Design review of the part built by this model. Coordinates are the model's own, in mm. A direction names the side the tool comes from. Give positions to 0.01 mm unless a question says otherwise; leave off trailing zeros. Write each loop counter-clockwise with the first axis right and the second up, starting at its lowest first coordinate (ties: lowest second). Pieces come first, ordered by that corner, then holes. Notation, with made-up numbers: (-19, 48) -> (-5, 48) arc R31 cw to (-5, 73) -> close; hole circle Ø9 at (7.5, 42). An arc over 180 degrees is marked (long way). Use CSV: the item, a comma, the result in double quotes.
```python
from build123d import *

# Parameters (mm, degrees)
F0_W      = 100
F0_H      = 63
F1_DEPTH  = 50
F3_DEPTH  = 50.001
F4_W      = 40
F4_H      = 15
F5_DEPTH  = 50.001
F7_DEPTH  = 9
F8_R      = 5
F9_DEPTH  = 41.001
F10_W     = 12
F10_H     = 10
F10_H_2   = 40
F11_DEPTH = 63.001
F13_DEPTH = 187
F15_DEPTH = 100.001
F16_R     = 25
F17_DEPTH = 18
F18_R     = 10
F19_DEPTH = 5
F22_DEPTH = 42
F20_R     = 25
F23_DEPTH = 8
F25_DEPTH = 8
F26_W     = 40
F26_H     = 9
F27_DEPTH = 8.001
F28_R     = 5
F29_DEPTH = 63.001


# Not quite as in the source:
# - an extrude ends at something that could not be found from the text; its depth is read off the source's solid


with BuildPart() as f1:
    # F0 (on Right) → F1 (new body)
    with BuildSketch(Plane.YZ):
        with Locations((50, 31.5)):
            Rectangle(F0_W, F0_H)
    extrude(amount=F1_DEPTH)

    # F2 (on face) → F3 (cut, through all)
    with BuildSketch(Plane.YZ.offset(50)):
        with BuildLine():
            Line((62.353148703, 6.3160295987), (45, 0))
            Line((45, 0), (85, 0))
            Line((85, 0), (83.3356871933, 1.6643128067))
            ThreePointArc((83.3356871933, 1.6643128067), (73.5223438483, 7.0480973254), (62.353148703, 6.3160295987))
        make_face()
    extrude(amount=-F3_DEPTH, mode=Mode.SUBTRACT)

    # F4 (on face) → F5 (cut, through all)
    with BuildSketch(Plane.YZ.offset(50)):
        with Locations((80, 55.5)):
            Rectangle(F4_W, F4_H)
    extrude(amount=-F5_DEPTH, mode=Mode.SUBTRACT)

    # F6 (on face) → F7 (cut)
    with BuildSketch(Plane.YZ.offset(50)):
        with BuildLine():
            ThreePointArc((84.8013158464, 48), (81.2386876382, 41.9291527956), (80, 35))
            ThreePointArc((80, 35), (85.8578643763, 20.8578643763), (100, 15))
            Line((100, 15), (100, 48))
            Line((100, 48), (84.8013158464, 48))
        make_face()
        with BuildLine():
            Line((80, 48), (80, 35))
            ThreePointArc((80, 35), (81.2386876382, 41.9291527956), (84.8013158464, 48))
            Line((84.8013158464, 48), (80, 48))
        make_face()
    extrude(amount=-F7_DEPTH, mode=Mode.SUBTRACT)

    # F8 (on face) → F9 (cut, through all)
    with BuildSketch(Plane.YZ.offset(41)):
        with Locations((90, 37.2308082879)):
            Circle(F8_R)
    extrude(amount=-F9_DEPTH, mode=Mode.SUBTRACT)

    # F10 (on face) → F11 (cut, through all)
    with BuildSketch(Plane.XY.offset(63)):
        with Locations((6, 55)):
            Rectangle(F10_W, F10_H)
        with Locations((6, 80)):
            Rectangle(F10_W, F10_H_2)
    extrude(amount=-F11_DEPTH, mode=Mode.SUBTRACT)

    # F12 (on face) → F13 (cut, through all)
    with BuildSketch(Plane.XZ):
        Polygon((0, 63), (0, 45), (6.5514642168, 63), align=None)
    extrude(amount=F13_DEPTH, mode=Mode.SUBTRACT)

    # F14 (on face) → F15 (cut, through all)
    with BuildSketch(Plane.XZ):
        Polygon((0, 63), (0, 45), (6.5514642168, 63), align=None)
    extrude(amount=-F15_DEPTH, mode=Mode.SUBTRACT)

    # F16 (on face) → F17 (cut)
    with BuildSketch(Plane.YZ.offset(50)):
        with Locations((30, 35)):
            Circle(F16_R)
    extrude(amount=-F17_DEPTH, mode=Mode.SUBTRACT)

    # F18 (on face) → F19 (join)
    with BuildSketch(Plane.YZ.offset(32)):
        with Locations((30, 35)):
            Circle(F18_R)
    extrude(amount=F19_DEPTH)

    # F21 (on face) → F22 (cut)
    with BuildSketch(Plane(origin=(0, 0, 0), x_dir=(0, -1, 0), z_dir=(-1, 0, 0))):
        with BuildLine():
            Line((-30, 63), (-30, 35))
            ThreePointArc((-30, 35), (21.9316580473, 14.5304524892), (-2.0665083135, 64.9287410926))
            Line((-2.0665083135, 64.9287410926), (-30, 63))
        make_face()
    extrude(amount=-F22_DEPTH, mode=Mode.SUBTRACT)

    # F20 (on face) → F23 (cut)
    with BuildSketch(Plane.YZ.offset(50)):
        with Locations((0, 35)):
            Circle(F20_R)
    extrude(amount=-F23_DEPTH, mode=Mode.SUBTRACT)

    # F24 (on face) → F25 (join)
    with BuildSketch(Plane.YZ.offset(37)):
        with BuildLine():
            ThreePointArc((29.5833333333, 30.017391357), (33.3850160019, 31.320099639), (35, 35))
            ThreePointArc((35, 35), (33.5355339059, 38.5355339059), (30, 40))
            Line((30, 40), (30, 35))
            ThreePointArc((30, 35), (29.8956518578, 32.5), (29.5833333333, 30.017391357))
        make_face()
        with BuildLine():
            Line((30, 35), (30, 40))
            ThreePointArc((30, 40), (25.0043497313, 35.2085147299), (29.5833333333, 30.017391357))
            ThreePointArc((29.5833333333, 30.017391357), (29.8956518578, 32.5), (30, 35))
        make_face()
    extrude(amount=F25_DEPTH)

    # F26 (on face) → F27 (cut, through all)
    with BuildSketch(Plane(origin=(42, 0, 0), x_dir=(0, -1, 0), z_dir=(-1, 0, 0))):
        with Locations((-10, 58.5)):
            Rectangle(F26_W, F26_H)
    extrude(amount=-F27_DEPTH, mode=Mode.SUBTRACT)

    # F28 (on face) → F29 (cut, through all)
    with BuildSketch(Plane.XY.offset(63)):
        with Locations((20, 39)):
            Circle(F28_R)
    extrude(amount=-F29_DEPTH, mode=Mode.SUBTRACT)


solid = f1.part
```
(1) Take a section at D-D (x = 29). Write out the cut boundary in (y, z).
Established:
outline,"(0, 0) -> (45, 0) -> (62.35, 6.32) arc R20 cw to (83.34, 1.66) -> (85, 0) -> (100, 0) -> (100, 48) -> (60, 48) -> (60, 63) -> (30, 63) -> (30, 35) arc R30 cw to (0, 5) -> close; hole circle Ø10 at (90, 37.23)"
(2) Take a section at A-A (x = 20). Write out the cut boundary in (y, z).
Established:
outline,"(0, 0) -> (34, 0) -> (34, 63) -> (30, 63) -> (30, 35) arc R30 cw to (0, 5) -> close; (44, 0) -> (45, 0) -> (62.35, 6.32) arc R20 cw to (83.34, 1.66) -> (85, 0) -> (100, 0) -> (100, 48) -> (60, 48) -> (60, 63) -> (44, 63) -> close; hole circle Ø10 at (90, 37.23)"
(3) Tool access review of faces 4 (the face through (45.563, 85.703, 21.014)), 5 (the face through (6, 50, 33)), 6 (the face through (42, 10, 9)), 7 (the face through (31, 60, 55)), 8 (the face through (37, 35.4, 35.1)): name each direction out of +Z, -Z, +X, -X, +Y, -Y from which nothing blocks a thin tool from reaching the whole face with its end or side.
Established:
face 4,"+Z, +X, +Y"
face 5,"+Z, -Z, -X, +Y"
face 6,"+Z, -X, -Y"
face 7,"+Z, +X, -X, +Y"
face 8,"+X"
(4) Mouldability with a two-part tool opening along Y and no side actions: class faces 1 (the face through (41.13, 53.5, 26.47)), 2 (the face through (3.23, 39.86, 53.87)), 3 (the face through (25, 0, 3)) as +Y half, -Y half, draft (parallel to the pull), parting line (faces both ways), or undercut.
Established:
face 1,"undercut"
face 2,"draft"
face 3,"-Y half"
(5) For line 1 along Y through (x, z) = (20, 40); line 2 along X through (y, z) = (56, 60); line 3 along Z through (x, y) = (27.75, 90), list the stretches that pass through material, from the lowest coordinate up. Write a range as [from, to].
Established:
line 1,"y = [30, 34], [44, 85.84], [94.16, 100]"
line 2,"x = [12, 50]"
line 3,"z = [0, 32.23], [42.23, 48]"
(6) Take a section at C-C (z = 27). Write out the cut boundary in (x, y).
Established:
outline,"(0, 28.91) -> (37, 28.91) -> (37, 36) -> (32, 36) -> (32, 53.69) -> (50, 53.69) -> (50, 81.67) -> (41, 81.67) -> (41, 100) -> (12, 100) -> (12, 50) -> (0, 50) -> close; hole circle Ø10 at (20, 39)"
(7) Clearance check with flat-ended pins moving along their axes: pin 1 (9.5 mm diameter, centred on x = 6.5, z = 31, fed in from +Y); pin 2 (10.5 mm diameter, centred on y = 33, z = 30.5, fed in from +X); pin 3 (2 mm diameter, centred on x = 38.5, y = 57, fed in from -Z). State where each tip first meets the part, or that it passes through.
Established:
pin 1,"stops at y = 50"
pin 2,"stops at x = 45"
pin 3,"stops at z = 4"
(8) Take a section at B-B (y = 90). Write out the cut boundary in (x, z), then the cut area to 3 significant figures.
Established:
outline,"(12, 0) -> (50, 0) -> (50, 17.68) -> (41, 17.68) -> (41, 32.23) -> (12, 32.23) -> close; (12, 42.23) -> (41, 42.23) -> (41, 48) -> (12, 48) -> close"
area,"1,260 mm2"
